Autodesk Inventor part; units mm, degrees
ref_plane "YZ Plane" through (0, 0, 0) normal (1, 0, 0) x (0, 1, 0)
ref_plane "XZ Plane" through (0, 0, 0) normal (0, 1, 0) x (-1, 0, 0)
ref_plane "XY Plane" through (0, 0, 0) normal (0, 0, 1) x (1, 0, 0)
sketch "Sketch1" plane through (0, 0, 0) normal (0, 1, 0) x (-1, 0, 0)
  line L0 (1.6166, 2.8) -> (3.2332, 0)
  line L1 (3.2332, 0) -> (1.6166, -2.8)
  line L2 (1.6166, -2.8) -> (-1.6166, -2.8)
  line L3 (-1.6166, -2.8) -> (-3.2332, 0)
  line L4 (-3.2332, 0) -> (-1.6166, 2.8)
  line L5 (-1.6166, 2.8) -> (1.6166, 2.8)
  line L6 (5.25, -4) -> (-5.25, -4)
  line L7 (-5.25, -4) -> (-5.25, 4)
  line L8 (-5.25, 4) -> (5.25, 4)
  line L9 (5.25, 4) -> (5.25, -4)
  line L10 (5.25, -4) -> (-5.25, 4) construction
  line L11 (-5.25, -4) -> (5.25, 4) construction
  point P0 (0, 0)
  point P1 (0, 0)
  point P2 (0, 0)
  dimension "d1" = 5.6
  dimension "d2" = 10.5
  dimension "d3" = 8
extrude "Extrusion1" add sketch "Sketch1" along normal blind 1.2 contours L0 L1 L2 L3 L4 L5 | L6 L7 L8 L9
sketch "Sketch2" plane through (-5.25, 0, 4) normal (0, 0, 1) x (1, 0, 0)
  line L0 (0, 0) -> (10.5, 0)
  line L1 (0, 0) -> (3, -3)
  line L2 (3, -3) -> (7.5, -3)
  line L3 (7.5, -3) -> (10.5, 0)
  point P0 (5.25, -3)
  point P1 (5.25, 0)
  dimension "d6" = 45
  dimension "d7" = 3
extrude "Extrusion2" add sketch "Sketch2" against normal up to surface (8 mm away)
extrude "Extrusion3" cut sketch "Sketch1" against normal up to surface (3 mm away) contours L0 L1 L2 L3 L4 L5
fillet "Fillet1" radius 1 6 edges at (5.25, 0, 0) (-5.25, 0, 0) (-2.25, -3, 2.8514) (2.25, -3, 2.8514) (2.25, -3, -2.8514) (-2.25, -3, -2.8514)
fillet "Fillet2" radius 1 18 edges at (2.2185, -2.9239, 4) (3.75, -1.5, 4) (5.1739, 0.0315, 4) (5.25, 0.8071, 4) (-2.2185, -2.9239, 4) (-3.75, -1.5, 4) (-5.1739, 0.0315, 4) (-5.25, 0.8071, 4) (0, -3, 4) (2.2185, -2.9239, -4) (3.75, -1.5, -4) (5.1739, 0.0315, -4) (5.25, 0.8071, -4) (-2.2185, -2.9239, -4) (-3.75, -1.5, -4) (-5.1739, 0.0315, -4) (-5.25, 0.8071, -4) (0, -3, -4)
hole "Hole1" at (0, 0, 0) direction (0, 1, 0) diameter 3.4036 end through all
properties part number "T Nut Adapter"
For this review, take the finished solid that the model builds, in its own axes (mm). A direction names the side the tool comes from. Coordinates: 2 decimals unless noted, no trailing zeros. Order: outer loops, then holes, each group sorted by start corner. A loop starts at its lowest first (then second) coordinate and runs counter-clockwise, first axis right, second up. Notation, with made-up numbers: (60, 73) - (111, 73) arc R24 ccw to (111, 87) - close; hole circle Ø5 at (32, 5). An arc over 180 degrees is marked (long way). Answer as a JSON object with one key per item and string values. Group by question number.
1. We need section B-B on y = 0.95. State the section outline as (x, z) points.
2. We need section A-A on x = 0. State the section outline as (y, z) points.
3. For probe 1 along Z at (x, y) = (0, 0.35); probe 2 along Z at (x, y) = (-1.25, -0.05); probe 3 along X at (y, z) = (0.5, 0), list the stretches that pass through material, from the lowest coordinate up.
4. We need section D-D on z = 2. State the section outline as (x, y) points, then the cut area to 3 significant figures.
5. We need section C-C on z = 0.75. State the section outline as (x, y) points, then the cut area to 3 significant figures.
6. Clearance check with flat-ended pins moving along their axes: P1, Ø3, axis at x = 0, z = 0, coming from the -Y side; P2, Ø1.5, axis at y = -2.5, z = -3, coming from the -X side; P3, Ø1.5, axis at x = -4, y = -2, coming from the -Z side. State where each tip first meets the part, or that it passes through.
7. For faces 1 (the flat face through (2.414, -1.479, -1.42)), 2 (the flat face through (0, 0, 4)), list the 3-axis set-ups (+Z, -Z, +X, -X, +Y, -Y) from which the entire face can be reached by the end or side of a thin tool; tool diameter is ignored.
Final values:
{
 "1": {"outline": "(-5.25, -3) arc R1 ccw to (-4.25, -4) - (4.25, -4) arc R1 ccw to (5.25, -3) - (5.25, 3) arc R1 ccw to (4.25, 4) - (-4.25, 4) arc R1 ccw to (-5.25, 3) - close; hole circle Ø3.4 at (0, 0)"},
 "2": {"outline": "(-3, -3) arc R1 ccw to (-2, -4) - (1.2, -4) - (1.2, -1.7) - (0, -1.7) - (0, -2.8) - (-3, -2.8) - close; (-3, 2.8) - (0, 2.8) - (0, 1.7) - (1.2, 1.7) - (1.2, 4) - (-2, 4) arc R1 ccw to (-3, 3) - close"},
 "3": {"probe 1": "-4 to -1.7, 1.7 to 4", "probe 2": "-4 to -2.8, 2.8 to 4", "probe 3": "-5.25 to -1.7, 1.7 to 5.25"},
 "4": {"outline": "(-5.25, 0.41) arc R1 ccw to (-4.96, -0.29) - (-2.54, -2.71) arc R1 ccw to (-2.08, -2.97) - (-2.08, 0) - (2.08, 0) - (2.08, -2.97) arc R1 ccw to (2.54, -2.71) - (4.96, -0.29) arc R1 ccw to (5.25, 0.41) - (5.25, 1.2) - (-5.25, 1.2) - close", "area": "22.5 mm²"},
 "5": {"outline": "(-5.25, 0.41) arc R1 ccw to (-4.96, -0.29) - (-2.8, -2.45) - (-2.8, 0) - (-1.53, 0) - (-1.53, 1.2) - (-5.25, 1.2) - close; (1.53, 0) - (2.8, 0) - (2.8, -2.45) - (4.96, -0.29) arc R1 ccw to (5.25, 0.41) - (5.25, 1.2) - (1.53, 1.2) - close", "area": "14.9 mm²"},
 "6": {"P1": "through", "P2": "x = -3.5", "P3": "z = -3.63"},
 "7": {"face 1": "-Y", "face 2": "+Z, +X, -X, +Y, -Y"}
}
